Verification items for the finished model (mm, model axes). Face numbers are marked on the shaded views. Give positions to 0.01 mm unless a question says otherwise; leave off trailing zeros. Put each result on its own line as item: value. Start each with the question number.
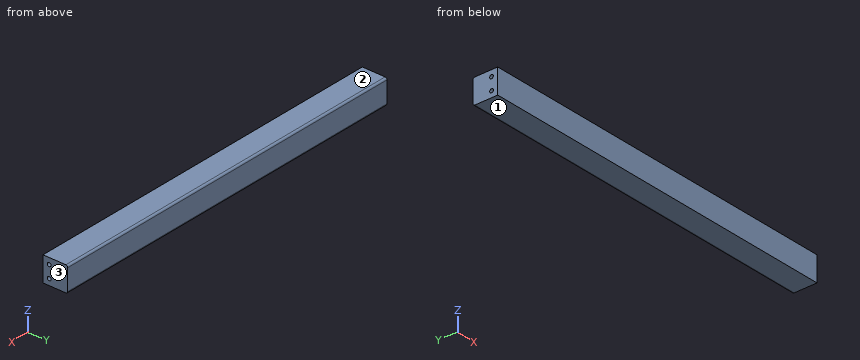
from build123d import *

# Parameters (mm, degrees)
SALIENTE_EXTRUIR1_DEPTH = 300
CROQUIS2_R              = 3
CORTAR_EXTRUIR1_DEPTH   = 10


with BuildPart() as part:
    # Croquis1 → Saliente-Extruir1 (new, symmetric)
    with BuildSketch(Plane(origin=(0, 0, 0), x_dir=(0, 0, -1), z_dir=(1, 0, 0))):
        with BuildLine():
            Line((20, -20), (-20, -20))
            Line((-20, -20), (-20, 17))
            ThreePointArc((-20, 17), (-19.121320344, 19.121320344), (-17, 20))
            Line((-17, 20), (17, 20))
            ThreePointArc((17, 20), (19.121320344, 19.121320344), (20, 17))
            Line((20, 17), (20, -20))
        make_face()
    extrude(amount=SALIENTE_EXTRUIR1_DEPTH, both=True)

    # Croquis2 → Cortar-Extruir1 (cut)
    with BuildSketch(Plane.ZY.offset(300)):
        with Locations((-10, -10)):
            Circle(CROQUIS2_R)
        with Locations((10, -10)):
            Circle(CROQUIS2_R)
    cortar_extruir1 = extrude(amount=-CORTAR_EXTRUIR1_DEPTH, mode=Mode.SUBTRACT)

    # Simetría1: Cortar-Extruir1 across plane
    add(cortar_extruir1.mirror(Plane(origin=(0, 0, 0), x_dir=(0, 0, 1), z_dir=(1, 0, 0))), mode=Mode.SUBTRACT)


solid = part.part
Q1. Release check for a two-part mould opening along Z. For the marked faces 1, 2 and 3 record: pulls with the +Z half, pulls with the -Z half, needs draft (parallel to the pull), parting line crosses it, or undercut.
Q2. Go/stop test with flat-tipped pins: pin 1 (1.8 mm diameter, centred on y = -9, z = 9, fed in from +X); pin 2 (3 mm diameter, centred on y = -10.5, z = -11, fed in from -X). Record where each tip stops, or that it passes through.
Q3. Scan lines: L1, parallel to Y at x = -292.5, z = -10; L2, parallel to X at y = -9, z = 10. Record each from-to range of solid material in increasing order.
Ans:
1. face 1: pulls with the -Z half
1. face 2: pulls with the +Z half
1. face 3: needs draft
2. pin 1: stops at x = 290
2. pin 2: stops at x = -290
3. L1: y = -20 to -13, -7 to 20
3. L2: x = -290 to 290
